```python
from build123d import *

# Parameters (mm, degrees)
ESBO_O1_W                = 90
ESBO_O1_H                = 70
RESSALTO_EXTRUS_O1_DEPTH = 2
RESSALTO_EXTRUS_O4_DEPTH = 8
ESBO_O6_W                = 66
ESBO_O6_H                = 15
CORTE_EXTRUS_O4_DEPTH    = 3
ESBO_O2_W                = 5.334
ESBO_O2_H                = 5.45
ESBO_O2_W_2              = 5.31
CORTE_EXTRUS_O6_DEPTH    = 5
ESBO_O7_R                = 1.6
CORTE_EXTRUS_O7_DEPTH    = 3


with BuildPart() as part:
    # Esboço1 → Ressalto-extrusão1 (new body)
    with BuildSketch(Plane(origin=(0, 0, 0), x_dir=(1, 0, 0), z_dir=(0, 1, 0))):
        Rectangle(ESBO_O1_W, ESBO_O1_H)
    extrude(amount=RESSALTO_EXTRUS_O1_DEPTH)

    # Esboço3 → Ressalto-extrusão4 (add)
    with BuildSketch(Plane(origin=(0, 2, 0), x_dir=(1, 0, 0), z_dir=(0, 1, 0))):
        Polygon((-35.8, -25.8), (-45, -25.8), (-45, -29.8), (-39.8, -29.8), (-39.8, -35), (-35.8, -35), align=None)
        Polygon((45, -29.8), (45, -25.8), (35.8, -25.8), (35.8, -35), (39.8, -35), (39.8, -29.8), align=None)
        Polygon((39.8, 35), (35.8, 35), (35.8, 25.8), (45, 25.8), (45, 29.8), (39.8, 29.8), align=None)
        Polygon((-35.8, 35), (-39.8, 35), (-39.8, 29.8), (-45, 29.8), (-45, 25.8), (-35.8, 25.8), align=None)
    extrude(amount=RESSALTO_EXTRUS_O4_DEPTH)

    # Esboço6 → Corte-extrusão4 (cut)
    with BuildSketch(Plane.XZ):
        with Locations((0, -22.5)):
            Rectangle(ESBO_O6_W, ESBO_O6_H)
    extrude(amount=-CORTE_EXTRUS_O4_DEPTH, mode=Mode.SUBTRACT)

    # Esboço2 → Corte-extrusão6 (cut)
    with BuildSketch(Plane(origin=(0, 2, 0), x_dir=(1, 0, 0), z_dir=(0, 1, 0))):
        with Locations((-37.333, -16.365)):
            Rectangle(ESBO_O2_W, ESBO_O2_H)
        with Locations((-37.333, -5.455)):
            Rectangle(ESBO_O2_W, ESBO_O2_H)
        with Locations((-26.663, -16.365)):
            Rectangle(ESBO_O2_W, ESBO_O2_H)
        with Locations((-26.663, -5.455)):
            Rectangle(ESBO_O2_W, ESBO_O2_H)
        with Locations((-15.993, -16.365)):
            Rectangle(ESBO_O2_W, ESBO_O2_H)
        with Locations((-15.993, -5.455)):
            Rectangle(ESBO_O2_W, ESBO_O2_H)
        with Locations((-5.323, -16.365)):
            Rectangle(ESBO_O2_W, ESBO_O2_H)
        with Locations((-5.323, -5.455)):
            Rectangle(ESBO_O2_W, ESBO_O2_H)
        with Locations((5.347, -16.365)):
            Rectangle(ESBO_O2_W, ESBO_O2_H)
        with Locations((5.347, -5.455)):
            Rectangle(ESBO_O2_W, ESBO_O2_H)
        with Locations((16.017, -16.365)):
            Rectangle(ESBO_O2_W, ESBO_O2_H)
        with Locations((16.017, -5.455)):
            Rectangle(ESBO_O2_W, ESBO_O2_H)
        with Locations((26.687, -16.365)):
            Rectangle(ESBO_O2_W, ESBO_O2_H)
        with Locations((26.687, -5.455)):
            Rectangle(ESBO_O2_W, ESBO_O2_H)
        with Locations((37.345, -16.365)):
            Rectangle(ESBO_O2_W_2, ESBO_O2_H)
        with Locations((37.345, -5.455)):
            Rectangle(ESBO_O2_W_2, ESBO_O2_H)
    extrude(amount=-CORTE_EXTRUS_O6_DEPTH, mode=Mode.SUBTRACT)

    # Esboço7 → Corte-extrusão7 (cut)
    with BuildSketch(Plane(origin=(0, 2, 0), x_dir=(1, 0, 0), z_dir=(0, 1, 0))):
        with Locations((31.5, 9)):
            Circle(ESBO_O7_R)
        with Locations((-5.5, 9)):
            Circle(ESBO_O7_R)
        with Locations((-5.5, -28)):
            Circle(ESBO_O7_R)
        with Locations((31.5, -28)):
            Circle(ESBO_O7_R)
    extrude(amount=-CORTE_EXTRUS_O7_DEPTH, mode=Mode.SUBTRACT)


solid = part.part
```
Could you check a few things on this model? Use its own coordinates, in mm. A direction names the side the tool comes from. Round coordinates to 2 decimals unless told otherwise and drop trailing zeros. Loops run counter-clockwise (first coordinate to the right, second up) from the corner with the lowest first, then second, coordinate; pieces in that order, holes last. Notation, with made-up numbers: (37, -32) - (94, -32) arc R8 cw to (94, -24) - close; hole circle Ø3 at (-5, 74.5). An arc over 180 degrees is marked (long way). Answer in a Markdown table with one row per item. Add a question column.
(1) If we section it at B-B (x = 31.5): Please give me the cut outline in (y, z).
(2) If we section it at C-C (x = -5.5): Please give me the cut outline in (y, z).
(3) I'm going to push flat-ended pins straight in: pin 1 (5.5 mm diameter, centred on x = -43.5, y = 7, fed in from -Z); pin 2 (12 mm diameter, centred on x = -24.5, z = 8.5, fed in from +Y); pin 3 (4 mm diameter, centred on y = 6, z = -33.5, fed in from -X). Where does each tip first touch, or does it pass through?
(4) If we mould it in two halves opening along X, with no side actions, what happens to faces 1 (the face through (-35.8, 6, 30)), 2 (the face through (-45, 1, 3)), 3 (the face through (-37, 1, 19.09)), 4 (the face through (-40, 6, 25.8))? For each: pulls with the +X half, pulls with the -X half, needs draft (parallel to the pull), parting line crosses it, or undercut.
(5) If we section it at A-A (z = -9): Please give me the cut outline in (x, y), plus the area to 3 significant figures.
(6) For faces 5 (the face through (35.8, 6, -30)), 6 (the face through (-27, 1, 19.09)), 7 (the face through (-42, 2, 32)), which set-ups out of +Z, -Z, +X, -X, +Y, -Y let a thin tool reach every point of the face, with its end or its side?
(7) I need wall thicknesses on line 1 along Z through (x, y) = (31.5, 0.6); line 2 along X through (y, z) = (0.45, -9); line 3 along X through (y, z) = (3, -29.5). Which ranges of each line are inside material? Lowest first, please.
(8) If we section it at D-D (z = -17): Please give me the cut outline in (x, y).
Model answer:
| question | item | result |
|---|---|---|
| 1 | outline | (0, -35) - (2, -35) - (2, -30) - (0, -30) - close; (0, -15) - (2, -15) - (2, -10.6) - (0, -10.6) - close; (0, -7.4) - (2, -7.4) - (2, 26.4) - (0, 26.4) - close; (0, 29.6) - (2, 29.6) - (2, 35) - (0, 35) - close |
| 2 | outline | (0, -35) - (2, -35) - (2, -30) - (0, -30) - close; (0, -15) - (2, -15) - (2, -10.6) - (0, -10.6) - close; (0, -7.4) - (2, -7.4) - (2, 2.73) - (0, 2.73) - close; (0, 8.18) - (2, 8.18) - (2, 13.64) - (0, 13.64) - close; (0, 19.09) - (2, 19.09) - (2, 26.4) - (0, 26.4) - close; (0, 29.6) - (2, 29.6) - (2, 35) - (0, 35) - close |
| 3 | pin 1 | stops at z = -29.8 |
| 3 | pin 2 | stops at y = 2 |
| 3 | pin 3 | stops at x = -39.8 |
| 4 | face 1 | undercut |
| 4 | face 2 | pulls with the -X half |
| 4 | face 3 | undercut |
| 4 | face 4 | needs draft |
| 5 | outline | (-45, 0) - (-7.1, 0) - (-7.1, 2) - (-45, 2) - close; (-3.9, 0) - (29.9, 0) - (29.9, 2) - (-3.9, 2) - close; (33.1, 0) - (45, 0) - (45, 2) - (33.1, 2) - close |
| 5 | area | 167 mm² |
| 6 | face 5 | +Z, -Z, +Y |
| 6 | face 6 | +Y, -Y |
| 6 | face 7 | +Z, -X, +Y |
| 7 | line 1 | z = -35 to -30, -15 to -10.6, -7.4 to 26.4, 29.6 to 35 |
| 7 | line 2 | x = -45 to -7.1, -3.9 to 29.9, 33.1 to 45 |
| 7 | line 3 | x = -45 to -35.8, 35.8 to 45 |
| 8 | outline | (-45, 0) - (-33, 0) - (-33, 2) - (-45, 2) - close; (33, 0) - (45, 0) - (45, 2) - (33, 2) - close |
